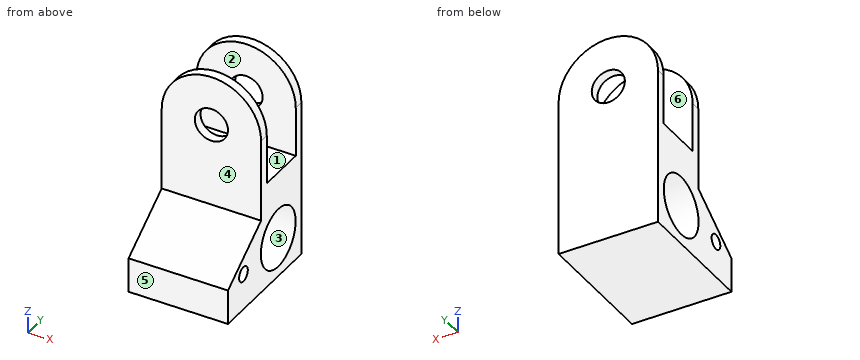
Autodesk Inventor part; units mm, degrees
ref_plane "YZ Plane" through (0, 0, 0) normal (1, 0, 0) x (0, 1, 0)
ref_plane "XZ Plane" through (0, 0, 0) normal (0, 1, 0) x (-1, 0, 0)
ref_plane "XY Plane" through (0, 0, 0) normal (0, 0, 1) x (1, 0, 0)
sketch "草圖1" plane through (0, 0, 0) normal (1, 0, 0) x (0, 1, 0)
  circle A0 centre (212.2024, 875) radius 90
  line L0 (152.2024, 1000) -> (352.2024, 1000)
  line L1 (352.2024, 1000) -> (352.2024, 785)
  circle A1 centre (32.2024, 865) radius 22.5
  line L2 (-154.9405, 785) -> (152.2024, 1000)
  line L3 (352.2024, 735) -> (352.2024, 1000)
  line L4 (-226.369, 735) -> (352.2024, 735)
  line L5 (152.2024, 1000) -> (-226.369, 735)
  line L6 (123.631, 980) -> (332.2024, 980)
  line L7 (332.2024, 980) -> (332.2024, 755)
  line L8 (332.2024, 755) -> (-47.7976, 755)
  line L9 (-47.7976, 755) -> (-47.7976, 860)
  line L10 (-47.7976, 860) -> (123.631, 980)
  circle A2 centre (212.2024, 875) radius 90
  circle A3 centre (32.2024, 865) radius 22.5
  point P0 (0, 0)
  dimension "d8" = 20
  dimension "d9" = 20
  dimension "d10" = 20
  dimension "d11" = 400
extrude "擠出1" add sketch "草圖1" along normal mid plane 300 contours L6 L7 L8 L9 L2
sketch "草圖2" plane through (-150, 332.2024, 980) normal (0, 1, 0) x (1, 0, 0)
  line L0 (0, 0) -> (300, 0)
  line L1 (300, 225) -> (300, 0)
  line L2 (300, 225) -> (0, 225)
  line L3 (0, 0) -> (0, 225)
  circle A0 centre (150, -250) radius 50
  circle A1 centre (150, -250) radius 150
  line L4 (0, 0) -> (300, 0)
  line L5 (0, 0) -> (0, -250)
  line L6 (300, 225) -> (300, 0)
  line L7 (300, 0) -> (300, -250)
  point P0 (150, 980)
  point P1 (150, 0)
  dimension "d14" = 250
  dimension "d15" = 100
extrude "擠出2" add sketch "草圖2" against normal blind 208.571 contours L0 L7 A1 L5 | A1
sketch "草圖3" plane through (150, 0, 0) normal (1, 0, 0) x (0, 0, -1)
  line L0 (-1230, 332.2024) -> (-1230, 332.2024)
  line L1 (-1230, 332.2024) -> (-1230, 123.6314)
  line L2 (-1230, 123.6314) -> (-1230, 123.6314)
  line L3 (-1230, 332.2024) -> (-1230, 123.6314)
  line L4 (-755, 332.2024) -> (-1230, 332.2024)
  line L5 (-1230, 332.2024) -> (-1230, 123.6314)
  line L6 (-980, 123.6314) -> (-1230, 123.6314)
  line L7 (-980, 123.6314) -> (-980, 123.631)
  line L8 (-980, 123.631) -> (-860, -47.7976)
  line L9 (-860, -47.7976) -> (-755, -47.7976)
  line L10 (-755, -47.7976) -> (-755, 332.2024)
  circle A0 centre (-875, 212.2024) radius 90
  circle A1 centre (-865, 32.2024) radius 22.5
  line L11 (-1380, 302.9169) -> (-1080, 302.9169)
  line L12 (-1080, 302.9169) -> (-1080, 152.9169)
  line L13 (-1080, 152.9169) -> (-1380, 152.9169)
  line L14 (-1380, 152.9169) -> (-1380, 302.9169)
  line L15 (-1380, 332.2024) -> (-1380, 123.6314)
  line L16 (-1380, 123.6314) -> (-1230, 123.6314)
  line L17 (-1230, 332.2024) -> (-1380, 332.2024)
  point P0 (0, 0)
  point P1 (-1380, 227.9169)
  point P2 (-1230, 227.9169)
  dimension "d18" = 150
  dimension "d19" = 300
extrude "擠出3" cut sketch "草圖3" against normal through all contours L11 L12 L13 L1 | L1 L13 L14 L11
thread "螺紋1"
sketch "草圖4" plane through (150, 152.9169, 1230) normal (0, 1, 0) x (1, 0, 0)
  line L0 (0, 150) -> (-300, 150)
  line L1 (-300, 0) -> (-300, 150)
  arc A0 (-300, 0) -> (0, 0) centre (-150, 0) ccw
  line L2 (0, 150) -> (0, 0)
  line L3 (0, 287.2857) -> (0, 150)
  line L4 (-300, 287.2857) -> (0, 287.2857)
  line L5 (-300, 150) -> (-300, 287.2857)
  line L6 (-300, 422.7143) -> (-300, 475)
  line L7 (-300, 475) -> (0, 475)
  line L8 (0, 475) -> (0, 422.7143)
  line L9 (0, 422.7143) -> (-300, 422.7143)
  circle A1 centre (-150, 0) radius 50
  point P0 (-150, 1230)
properties part number "萬象塊"
Design review of the part built by this model. Coordinates are the model's own, in mm. Face numbers are marked on the shaded views. A direction names the side the tool comes from. Coordinates: 2 decimals unless noted, no trailing zeros. Write each loop counter-clockwise with the first axis right and the second up, starting at its lowest first coordinate (ties: lowest second). Pieces come first, ordered by that corner, then holes.
1) Add section C-C (x = 9). State how many separate pieces and enclosed holes the cut face has, plus the area to 3 significant figures.
2) Add section B-B (y = 131.5). Write out the cut boundary in (x, z).
3) Insertion check: pin 1 (1.5 mm diameter, centred on x = 58.5, z = 1172.5, fed in from -Y); pin 2 (3 mm diameter, centred on x = 70, y = 52, fed in from +Z). Each pin has a flat end and moves straight along its axis. Give the tip position at first contact, or say it passes through.
4) Mouldability with a two-part tool opening along Z and no side actions: class the marked faces 1, 2 and 3 as +Z half, -Z half, draft (parallel to the pull), parting line (faces both ways), or undercut.
5) To check wall thickness, follow L1, parallel to X at y = 144, z = 1230; L2, parallel to Z at x = 36, y = 132.5; L3, parallel to Y at x = 54, z = 1148.5. State the ranges of each line that lie inside material, in increasing order.
6) Add section A-A (z = 1153.5). Write out the cut boundary in (x, y).
7) Add section D-D (z = 875). Write out the cut boundary in (x, y), plus the area to 3 significant figures.
8) Machinability: for the marked faces 4, 5 and 6, which of the approach directions +Z, -Z, +X, -X, +Y, -Y give a long, thin tool a straight path to every point of the face, cutting with its end or side? Answer none if there is none.
Check result:
1. separate pieces: 3
1. enclosed holes: 2
1. area: 80,800 mm2
2. outline: (-150, 755) - (150, 755) - (150, 835.16) - (-150, 835.16) - close; (-150, 914.84) - (150, 914.84) - (150, 1230) arc R150 ccw to (-150, 1230) - close; hole circle Ø100 at (0, 1230)
3. pin 1: stops at y = 123.63
3. pin 2: stops at z = 930.91
4. face 1: +Z half
4. face 2: draft
4. face 3: undercut
5. L1: x = -150 to -50, 50 to 150
5. L2: z = 755 to 833.2, 916.8 to 1195.3, 1264.7 to 1375.62
5. L3: y = 123.63 to 152.92, 302.92 to 332.2
6. outline: (-150, 123.63) - (150, 123.63) - (150, 152.92) - (-150, 152.92) - close; (-150, 302.92) - (150, 302.92) - (150, 332.2) - (-150, 332.2) - close
7. outline: (-150, -26.37) - (150, -26.37) - (150, 12.05) - (-150, 12.05) - close; (-150, 52.36) - (150, 52.36) - (150, 122.2) - (-150, 122.2) - close; (-150, 302.2) - (150, 302.2) - (150, 332.2) - (-150, 332.2) - close
7. area: 41,500 mm2
8. face 4: +Z, +X, -X, -Y
8. face 5: +Z, -Z, +X, -X, -Y
8. face 6: +Z, +X, -X
